Check sheet for the modelled part. Datum: model origin and axes. Units: mm. A direction names the side the tool comes from. Coordinates: 2 decimals unless noted, no trailing zeros. Loops run counter-clockwise (first coordinate to the right, second up) from the corner with the lowest first, then second, coordinate; pieces in that order, holes last. Notation, with made-up numbers: M 48.25,-36 L 53.25,-36 A15 cw 53.25,-25 Z; hole C -12.75,-31.75 d7. An arc over 180 degrees is marked long. Return JSON: item names as keys, results as strings.
from build123d import *

# Parameters (mm, degrees)
F0_R     = 19.05
F1_DEPTH = 31.75
F4_R     = 25.4
F5_DEPTH = 5.08
F3_R     = 12.7
F6_DEPTH = 30.48
F2_R     = 10.16
F7_DEPTH = 42.672
F8_DEPTH = 5.08


with BuildPart() as f1:
    # F0 (on Top) → F1 (new body)
    with BuildSketch(Plane.XY):
        Circle(F0_R)
    extrude(amount=F1_DEPTH)

    # F4 (on face) → F5 (join)
    with BuildSketch(Plane.XY.offset(31.75)):
        Circle(F4_R)
    extrude(amount=-F5_DEPTH)

    # F3 (on face) → F6 (cut)
    with BuildSketch(Plane(origin=(0, 0, 0), x_dir=(1, 0, 0), z_dir=(0, 0, -1))):
        Circle(F3_R)
    extrude(amount=-F6_DEPTH, mode=Mode.SUBTRACT)

    # F2 (on face) → F7 (cut)
    with BuildSketch(Plane(origin=(0, 0, 0), x_dir=(1, 0, 0), z_dir=(0, 0, -1))):
        Circle(F2_R)
    extrude(amount=-F7_DEPTH, mode=Mode.SUBTRACT)

    # F8 (add): a face of the model
    f8_faces = [f1.faces().sort_by_distance(p)[0] for p in [
        (-18.5111846327, 0, 0),
    ]]
    extrude(f8_faces, amount=F8_DEPTH)


solid = f1.part
1) Go/stop test with flat-tipped pins: pin 1 Ø8 at (y, z) = (-15.5, 26) entering from -X; pin 2 Ø1 at (x, z) = (-2, 9) entering from +Y; pin 3 Ø4 at (y, z) = (13.5, 5.5) entering from +X; pin 4 Ø16.5 at (x, y) = (0, 0) entering from -Z. Record where each tip stops, or that it passes through.
Answers:
{"pin 1": "x = -22.62", "pin 2": "y = 18.99", "pin 3": "x = 15.19", "pin 4": "through"}
2) Draft check along Y on faces 3 (the face through (-6, -9, 30.48)), 4 (the face through (-5.506, -24.796, 29.246)), 5 (the face through (4, -12.4, -5.08)). Enter one of: +Y half, -Y half, draft (parallel to the pull), parting line (faces both ways), or undercut.
Answers:
{"face 3": "undercut", "face 4": "parting line", "face 5": "draft"}
3) Set-up check for faces 1 (the face through (4, 19, 26.67)), 2 (the face through (-1.323, -10.074, 31.106)): record each of +Z, -Z, +X, -X, +Y, -Y from which the full face is reachable in a straight line by a thin tool's end or side.
Answers:
{"face 1": "-Z", "face 2": "+Z, -Z"}
4) Section check C-C on z = 12. Record the cut outline in (x, y).
Answers:
{"outline": "C 0,0 d38.1; hole C 0,0 d25.4"}
5) Section check D-D on x = 22.5. Record the cut outline in (y, z).
Answers:
{"outline": "M -11.79,26.67 L 11.79,26.67 L 11.79,31.75 L -11.79,31.75 Z"}
6) Scan lines: line 1 along Y through (x, z) = (0, 31.4); line 2 along Y through (x, z) = (0, 21); line 3 along Z through (x, y) = (-19, -3). Record each from-to range of solid material in increasing order. Write a range as [from, to].
Answers:
{"line 1": "[-25.4, -10.16], [10.16, 25.4]", "line 2": "[-19.05, -12.7], [12.7, 19.05]", "line 3": "[26.67, 31.75]"}
7) Section check A-A on x = 0. Record the cut outline in (y, z).
Answers:
{"outline": "M -25.4,26.67 L -19.05,26.67 L -19.05,-5.08 L -12.7,-5.08 L -12.7,30.48 L -10.16,30.48 L -10.16,31.75 L -25.4,31.75 Z; M 10.16,30.48 L 12.7,30.48 L 12.7,-5.08 L 19.05,-5.08 L 19.05,26.67 L 25.4,26.67 L 25.4,31.75 L 10.16,31.75 Z"}
